Work out the finished part from the listing and answer in its coordinate system (mm). A direction names the side the tool comes from. Coordinates: 2 decimals unless noted, no trailing zeros. Order: outer loops, then holes, each group sorted by start corner. A loop starts at its lowest first (then second) coordinate and runs counter-clockwise, first axis right, second up. Notation, with made-up numbers: M 4,-33.5 L 62,-33.5 A36 cw 62,3.5 Z; hole C 0,-22 d9. An arc over 180 degrees is marked long. Write item = value, one per line. Start each with the question number.
Q1. Find section A-A on y = -0.75. Give the vertices of the cut face in (x, z).
Q2. A tool of negligible diameter and unlimited length cuts with its end or side. For faces 4 (the flat face through (-3.4, -13.5, 10)), 5 (the flat face through (-38.3, -5, 3.8)), 6 (the flat face through (38.3, -5, 3.8)), from which of +Z, -Z, +X, -X, +Y, -Y can it reach the whole face along a straight path? Write none if from no direction.
Q3. Find section B-B on x = -36.25. Give the vertices of the cut face in (y, z), and give its area (3 significant figures).
Q4. Determine the mould class of faces 1 (the flat face through (-43.75, -2, 5)), 2 (the flat face through (-3.4, -13.5, 0)), 3 (the cylindrical face through (-34.2, -2.54, 5.65)) for opening direction Z: released by +Z, released by -Z, zero draft, split by the parting line, or undercut.
Q5. Find section D-D on z = 9. Give the vertices of the cut face in (x, y).
Q6. Each of these flat-tipped pins is pushed along its axis until it touches: P1, Ø3, axis at x = 27.5, z = 3.5, coming from the +Y side; P2, Ø5, axis at x = 36.25, z = 5, coming from the -Y side; P3, Ø1, axis at x = -11, y = -5, coming from the +Z side; P4, Ø4, axis at x = -16, z = 3.5, coming from the -Y side. Where does it stop, or does it pass through?
Q7. Straight lines are drawn through the part: line 1 along Z through (x, y) = (36.25, -2.1); line 2 along Y through (x, z) = (-39, 6); line 3 along X through (y, z) = (-4, 7.75). For each, find the intervals that lie inside material, in ascending order.
Q8. Find section C-C on z = 5. Give the vertices of the cut face in (x, y), and give its area (3 significant figures).
Autodesk Inventor part; units mm, degrees
ref_plane "YZ Plane" through (0, 0, 0) normal (1, 0, 0) x (0, 1, 0)
ref_plane "XZ Plane" through (0, 0, 0) normal (0, 1, 0) x (-1, 0, 0)
ref_plane "XY Plane" through (0, 0, 0) normal (0, 0, 1) x (1, 0, 0)
sketch "Sketch1" plane through (0, 0, 0) normal (0, 0, 1) x (1, 0, 0)
  circle A0 centre (0, 0) radius 13.75
  circle A1 centre (0, 0) radius 18.75
  line L0 (-18.75, 0) -> (-43.75, 0)
  line L1 (-43.75, 0) -> (-43.75, -5)
  line L2 (-43.75, -5) -> (-18.75, -5)
  line L3 (-18.75, -5) -> (-18.75, 0)
  line L4 (-18.75, -5) -> (-13.75, -5)
  line L5 (-13.75, -5) -> (-13.75, 0)
  line L6 (-13.75, 0) -> (-18.75, 0)
  line L7 (-18.75, 0) -> (-18.75, -5)
  line L8 (18.75, 0) -> (43.75, 0)
  line L9 (43.75, 0) -> (43.75, -5)
  line L10 (43.75, -5) -> (18.75, -5)
  line L11 (18.75, -5) -> (18.75, 0)
  line L12 (18.75, -5) -> (13.75, -5)
  line L13 (13.75, -5) -> (13.75, 0)
  line L14 (13.75, 0) -> (18.75, 0)
  line L15 (18.75, 0) -> (18.75, -5)
  point P0 (-18.071, -5)
  point P1 (18.071, -5)
  dimension "d0" = 27.5
  dimension "d1" = 5
  dimension "d2" = 5
  dimension "d3" = 25
  dimension "d4" = 25
  dimension "d5" = 5
extrude "Extrusion1" add sketch "Sketch1" along normal blind 10 contours L13 L12 A1 L4 L5 A0 | L14 A1 L12 L13 | L5 L4 A1 L6 | L11 L12 A1 | L8 L9 L10 L11 | L3 L2 L1 L0 | A1 L4 L3
sketch "Sketch2" plane through (-43.75, -5, 0) normal (0, -1, 0) x (1, 0, 0)
  line L0 (0, 0) -> (25.679, 0)
  line L1 (25.679, 0) -> (25.679, 10)
  line L2 (0, 10) -> (25.679, 10)
  line L3 (0, 0) -> (0, 10)
  line L4 (61.821, 0) -> (87.5, 0)
  line L5 (87.5, 0) -> (87.5, 10)
  line L6 (61.821, 10) -> (87.5, 10)
  line L7 (61.821, 0) -> (61.821, 10)
  circle A0 centre (7.5, 5) radius 2.15
  circle A1 centre (80, 5) radius 2.15
  line L8 (0, 0) -> (0, 10)
  line L9 (87.5, 0) -> (87.5, 10)
  point P0 (43.75, 0)
  point P1 (12.8395, 10)
  point P2 (0, 5)
  point P3 (74.6605, 10)
  point P4 (87.5, 5)
  point P5 (0, 5)
  point P6 (0, 5)
  point P7 (87.5, 5)
  point P8 (87.5, 5)
  dimension "d8" = 4.3
  dimension "d9" = 4.3
  dimension "d13" = 7.5
  dimension "d14" = 7.5
extrude "Extrusion2" cut sketch "Sketch2" against normal up to surface (5 mm away) contours A0 | A1
fillet "Fillet1" radius 20 2 edges at (-18.071, -5, 5) (18.071, -5, 5)
equation "\"d4\" = d3"
Findings below:
q1.outline = M -43.75,0 L -13.73,0 L -13.73,10 L -43.75,10 Z; M 13.73,0 L 43.75,0 L 43.75,10 L 13.73,10 Z; hole C -36.25,5 d4.3; hole C 36.25,5 d4.3
q2.face_4 = +Z, +X, -X, +Y, -Y
q2.face_5 = +Z, -Z, -X, -Y
q2.face_6 = +Z, -Z, +X, -Y
q3.outline = M -5,0 L 0,0 L 0,2.85 L -5,2.85 Z; M -5,7.15 L 0,7.15 L 0,10 L -5,10 Z
q3.area = 28.5 mm^2
q4.face_1 = zero draft
q4.face_2 = released by -Z
q4.face_3 = undercut
q5.outline = M -43.75,-5 L -29.61,-5 A20 cw -14.33,-12.1 A18.75 ccw 14.33,-12.1 A20 cw 29.61,-5 L 43.75,-5 L 43.75,0 L 13.75,0 A13.75 cw -13.75,0 L -43.75,0 Z
q6.P1 = 0
q6.P2 = -5
q6.P3 = through
q6.P4 = -12.47
q7.line_1 = 0 to 2.85, 7.15 to 10
q7.line_2 = -5 to 0
q7.line_3 = -43.75 to -13.16, 13.16 to 43.75
q8.outline = M -43.75,-5 L -38.4,-5 L -38.4,0 L -43.75,0 Z; M -34.1,-5 L -29.61,-5 A20 cw -14.33,-12.1 A18.75 ccw 14.33,-12.1 A20 cw 29.61,-5 L 34.1,-5 L 34.1,0 L 13.75,0 A13.75 cw -13.75,0 L -34.1,0 Z; M 38.4,-5 L 43.75,-5 L 43.75,0 L 38.4,0 Z
q8.area = 500 mm^2
